Could you check a few things on this model? Use its own coordinates, in mm. A direction names the side the tool comes from. Round coordinates to 2 decimals unless told otherwise and drop trailing zeros. Loops run counter-clockwise (first coordinate to the right, second up) from the corner with the lowest first, then second, coordinate; pieces in that order, holes last.
from build123d import *

# Parameters (mm, degrees)
SKETCH2_R                = 7.5
BOSS_EXTRUDE4_DEPTH      = 5
BOSS_EXTRUDE5_DEPTH      = 1
BOSS_EXTRUDE5_DEPTH_BACK = 22
SKETCH5_R                = 7.5
CHAMFER1_SIZE            = 1
BOSS_EXTRUDE8_DEPTH      = 1
BOSS_EXTRUDE8_DEPTH_BACK = 22
SKETCH8_R                = 7.5
CHAMFER3_SIZE            = 1


with BuildPart() as part:
    # Sketch2 → Boss-Extrude4 (new, symmetric)
    with BuildSketch(Plane(origin=(0, 0, 0), x_dir=(1, 0, 0), z_dir=(0, 1, 0))):
        with BuildLine():
            Line((-141.647927202, 154.020874391), (399.122072798, 154.020874391))
            ThreePointArc((399.122072798, 154.020874391), (414.122072798, 139.020874391), (399.122072798, 124.020874391))
            Line((399.122072798, 124.020874391), (-141.647927202, 124.020874391))
            ThreePointArc((-141.647927202, 124.020874391), (-156.647927202, 139.020874391), (-141.647927202, 154.020874391))
        make_face()
        with Locations(Location((-141.647927202, 139.020874391, 0), (0, 0, 270))):
            Circle(SKETCH2_R, mode=Mode.SUBTRACT)
        with Locations(Location((399.122072798, 139.020874391, 0), (0, 0, 270))):
            Circle(SKETCH2_R, mode=Mode.SUBTRACT)
    extrude(amount=BOSS_EXTRUDE4_DEPTH, both=True)

    # Sketch5 → Boss-Extrude5 (add, two sides: drawn at the far end of the back side and taken through both)
    with BuildSketch(Plane(origin=(0, 5, 0), x_dir=(1, 0, 0), z_dir=(0, 1, 0)).offset(-BOSS_EXTRUDE5_DEPTH_BACK)):
        with Locations(Location((-141.647927202, 139.020874391, 0), (0, 0, 270))):
            Circle(SKETCH5_R)
    extrude(amount=BOSS_EXTRUDE5_DEPTH + BOSS_EXTRUDE5_DEPTH_BACK)

    # Chamfer1
    chamfer1_edges = [part.edges().sort_by_distance(p)[0] for p in [
        (-141.647927202, -17, -146.520874391),
    ]]
    chamfer(chamfer1_edges, length=CHAMFER1_SIZE)

    # Sketch8 → Boss-Extrude8 (add, two sides: drawn at the far end of the back side and taken through both)
    with BuildSketch(Plane(origin=(0, 5, 0), x_dir=(1, 0, 0), z_dir=(0, 1, 0)).offset(-BOSS_EXTRUDE8_DEPTH_BACK)):
        with Locations(Location((399.122072798, 139.020874391, 0), (0, 0, 270))):
            Circle(SKETCH8_R)
    extrude(amount=BOSS_EXTRUDE8_DEPTH + BOSS_EXTRUDE8_DEPTH_BACK)

    # Chamfer3
    chamfer3_edges = [part.edges().sort_by_distance(p)[0] for p in [
        (399.122072798, -17, -146.520874391),
    ]]
    chamfer(chamfer3_edges, length=CHAMFER3_SIZE)


solid = part.part
Item 1: If we section it at A-A, the plane y = -9: Please give me the cut outline in (x, z), then the cut area to 3 significant figures.
Results list:
outline: circle Ø15 at (-141.65, -139.02); circle Ø15 at (399.12, -139.02)
area: 353 mm2
Item 2: Will these pins go through, and if not, where does the flat tip stop? pin 1 (5 mm diameter, centred on y = -6, z = -133.5, fed in from -X); pin 2 (1.5 mm diameter, centred on x = 176, z = -138, fed in from +Y); pin 3 (1 mm diameter, centred on y = 0.5, z = -132, fed in from +X).
Results list:
pin 1: stops at x = -156.3
pin 2: stops at y = 5
pin 3: stops at x = 412.63
Item 3: If I drill on line 1 along Y through (x, z) = (26, -135.75); line 2 along X through (y, z) = (-3, -140.5); line 3 along X through (y, z) = (-15, -133), over which ranges is the centre line in solid material (lowest first)?
Results list:
line 1: y = -5 to 5
line 2: x = -156.57 to 414.05
line 3: x = -146.12 to -137.18, 394.65 to 403.59
Item 4: For faces 4 (the cylindrical face through (391.8, -10.58, -140.65)), 5 (the cylindrical face through (-156.644, 0.07, -138.691)), 6 (the cylindrical face through (-146.212, 5.493, -144.973)), which set-ups out of +Z, -Z, +X, -X, +Y, -Y let a thin tool reach every point of the face, with its end or its side?
Results list:
face 4: -Y
face 5: -X, +Y, -Y
face 6: +Y
Item 5: If we section it at B-B, the plane x = 275: Please give me the cut outline in (y, z), then the cut area to 3 significant figures.
Results list:
outline: (-5, -154.02) - (5, -154.02) - (5, -124.02) - (-5, -124.02) - close
area: 300 mm2
Item 6: We'd pull the mould along X, two halves only. Please class faces 1 (the cylindrical face through (414.12, 0.07, -139.35)), 2 (the flat face through (-142, -17, -139)), 3 (the cylindrical face through (-146.212, -10.577, -144.973)): released by +X, released by -X, zero draft, split by the parting line, or undercut.
Results list:
face 1: released by +X
face 2: zero draft
face 3: undercut
